The drawing under review shows one solid part. Ordinate dimensions are in mm from its lowest x, y, z. A direction names the side the tool comes from. Coordinates: 2 decimals unless noted, no trailing zeros. Write each loop counter-clockwise with the first axis right and the second up, starting at its lowest first coordinate (ties: lowest second). Pieces come first, ordered by that corner, then holes. Notation, with made-up numbers: (75.5, 53) - (113.5, 53) arc R29 ccw to (113.5, 90) - close; hole circle Ø4 at (78.5, 60). An arc over 180 degrees is marked (long way). Put each result on its own line as item: value. Start each with the question number.
Item 1: Mouldability with a two-part tool opening along X and no side actions: class the marked faces 3, 4, 5 and 6 as pulls with the +X half, pulls with the -X half, needs draft (parallel to the pull), parting line crosses it, or undercut.
Item 2: For pin 1 (5 mm diameter, centred on y = 4.5, z = 26, fed in from -X); pin 2 (8 mm diameter, centred on y = 5.5, z = 26, fed in from +X) (1 decimal); pin 3 (5 mm diameter, centred on x = 127.53, y = 15, fed in from -Z); pin 4 (9.5 mm diameter, centred on x = 37.5, y = 15, fed in from -Z), all flat-tipped, find the tip position at first contact; note any pin that passes through.
Item 3: Machinability: for the marked faces 1 and 2, which of the approach directions +Z, -Z, +X, -X, +Y, -Y give a long, thin tool a straight path to every point of the face, cutting with its end or side? Answer none if there is none.
Item 4: Consider section C-C on x = 15. Give the boundary of the cut face in (y, z).
Item 5: Consider section D-D on z = 13.5. Give the boundary of the cut face in (x, y), then the cut area to 3 significant figures.
Item 6: Consider section B-B on y = 15. Give the boundary of the cut face in (x, z), then the cut area to 3 significant figures.
Item 7: To check wall thickness, follow L1, parallel to Z at x = 20.5, y = 2; L2, parallel to Y at x = 37, z = 37; L3, parallel to Y at x = 37.5, z = 38.05. State the ranges of each line that lie inside material, in increasing order. Write a range as [from, to].
Item 8: Consider section A-A on x = 105. Give the boundary of the cut face in (y, z), then the cut area to 3 significant figures.
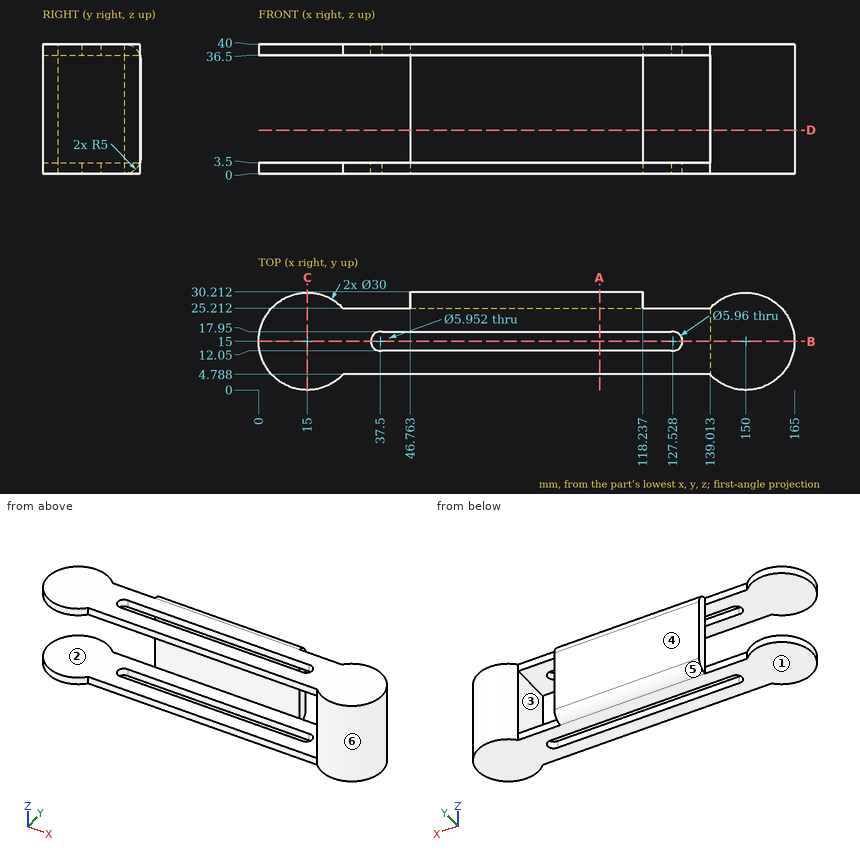
Report:
1. face 3: pulls with the -X half
1. face 4: needs draft
1. face 5: undercut
1. face 6: undercut
2. pin 1: x = 139.01
2. pin 2: x = 164
2. pin 3: through
2. pin 4: z = 0
3. face 1: -Z, +X, -X, +Y, -Y
3. face 2: -X, -Y
4. outline: (0, 0) - (30, 0) - (30, 3.5) - (0, 3.5) - close; (0, 36.5) - (30, 36.5) - (30, 40) - (0, 40) - close
5. outline: (46.76, 25.21) - (118.24, 25.21) - (118.24, 30.21) - (46.76, 30.21) - close; (139.01, 4.79) arc R15 ccw (long way) to (139.01, 25.21) - close
5. area: 1,010 mm²
6. outline: (0, 0) - (34.52, 0) - (34.52, 3.5) - (0, 3.5) - close; (0, 36.5) - (34.52, 36.5) - (34.52, 40) - (0, 40) - close; (130.51, 0) - (165, 0) - (165, 40) - (130.51, 40) - (130.51, 36.5) - (139.01, 36.5) - (139.01, 3.5) - (130.51, 3.5) - close
6. area: 1,340 mm²
7. L1: [0, 3.5], [36.5, 40]
7. L2: [4.79, 12.07], [17.93, 25.21]
7. L3: [4.79, 12.02], [17.98, 25.21]
8. outline: (4.79, 0) - (12.05, 0) - (12.05, 3.5) - (4.79, 3.5) - close; (4.79, 36.5) - (12.05, 36.5) - (12.05, 40) - (4.79, 40) - close; (17.95, 0) - (25.21, 0) arc R5 ccw to (30.21, 5) - (30.21, 35) arc R5 ccw to (25.21, 40) - (17.95, 40) - (17.95, 36.5) - (25.21, 36.5) - (25.21, 3.5) - (17.95, 3.5) - close
8. area: 291 mm²
